Check sheet for the modelled part. Datum: model origin and axes. Units: mm. Give positions to 0.01 mm unless a question says otherwise; leave off trailing zeros. Order: outer loops, then holes, each group sorted by start corner. A loop starts at its lowest first (then second) coordinate and runs counter-clockwise, first axis right, second up. Notation, with made-up numbers: (54, -21.75) -> (91, -21.75) arc R6 ccw to (91, -11.75) -> close; hole circle Ø8 at (-4.5, 64). An arc over 180 degrees is marked (long way). Answer in a Markdown table with one row per item. Add a question column.
(1) Release check for a two-part mould opening along Z. For faces 1 (the face through (37.8, 11.66, 25.12)), 2 (the face through (-41.64, 11.66, -27.1)), 3 (the face through (42.5, 11, 0)) record: released by +Z, released by -Z, zero draft, split by the parting line, or undercut.
(2) Thickness scan on L1, parallel to X at y = 7, z = 24.5. Record the ranges inside material, lowest first. Write a range as [from, to].
(3) Cross-section at A-A (x = -19). Record the cut outline in (y, z).
(4) Go/stop test with a flat-tipped pin: pin 1 (2.5 mm diameter, centred on x = 39, z = 24.5, fed in from -Y). Record where the tip stops, or that it passes through.
```python
from build123d import *

# Parameters (mm, degrees)
CROQUIS1_W              = 85
CROQUIS1_H              = 56
SALIENTE_EXTRUIR1_DEPTH = 23
REDONDEO1_R             = 3
CROQUIS2_R              = 1.35
CORTAR_EXTRUIR1_DEPTH   = 56.850246195


with BuildPart() as part:
    # Croquis1 → Saliente-Extruir1 (new body)
    with BuildSketch(Plane(origin=(0, 0, 0), x_dir=(1, 0, 0), z_dir=(0, 1, 0))):
        Rectangle(CROQUIS1_W, CROQUIS1_H)
    extrude(amount=SALIENTE_EXTRUIR1_DEPTH)

    # Redondeo1
    redondeo1_edges = [part.edges().sort_by_distance(p)[0] for p in [
        (-42.5, 11.5, -28),
        (42.5, 11.5, -28),
        (42.5, 11.5, 28),
        (-42.5, 11.5, 28),
    ]]
    fillet(redondeo1_edges, radius=REDONDEO1_R)

    # Croquis2 → Cortar-Extruir1 (cut, through all)
    with BuildSketch(Plane(origin=(0, 23, 0), x_dir=(1, 0, 0), z_dir=(0, 1, 0))):
        with Locations(Location((-19, 24.5, 0), (0, 0, 270))):
            Circle(CROQUIS2_R)
        with Locations(Location((39, 24.5, 0), (0, 0, 270))):
            Circle(CROQUIS2_R)
        with Locations(Location((39, -24.5, 0), (0, 0, 270))):
            Circle(CROQUIS2_R)
        with Locations(Location((-19, -24.5, 0), (0, 0, 270))):
            Circle(CROQUIS2_R)
    extrude(amount=-CORTAR_EXTRUIR1_DEPTH, mode=Mode.SUBTRACT)


solid = part.part
```
Answer below:
| question | item | result |
|---|---|---|
| 1 | face 1 | undercut |
| 1 | face 2 | released by -Z |
| 1 | face 3 | zero draft |
| 2 | L1 | x = [-42.5, -20.35], [-17.65, 37.65], [40.35, 42.5] |
| 3 | outline | (0, -28) -> (23, -28) -> (23, -25.85) -> (0, -25.85) -> close; (0, -23.15) -> (23, -23.15) -> (23, 23.15) -> (0, 23.15) -> close; (0, 25.85) -> (23, 25.85) -> (23, 28) -> (0, 28) -> close |
| 4 | pin 1 | passes through |
